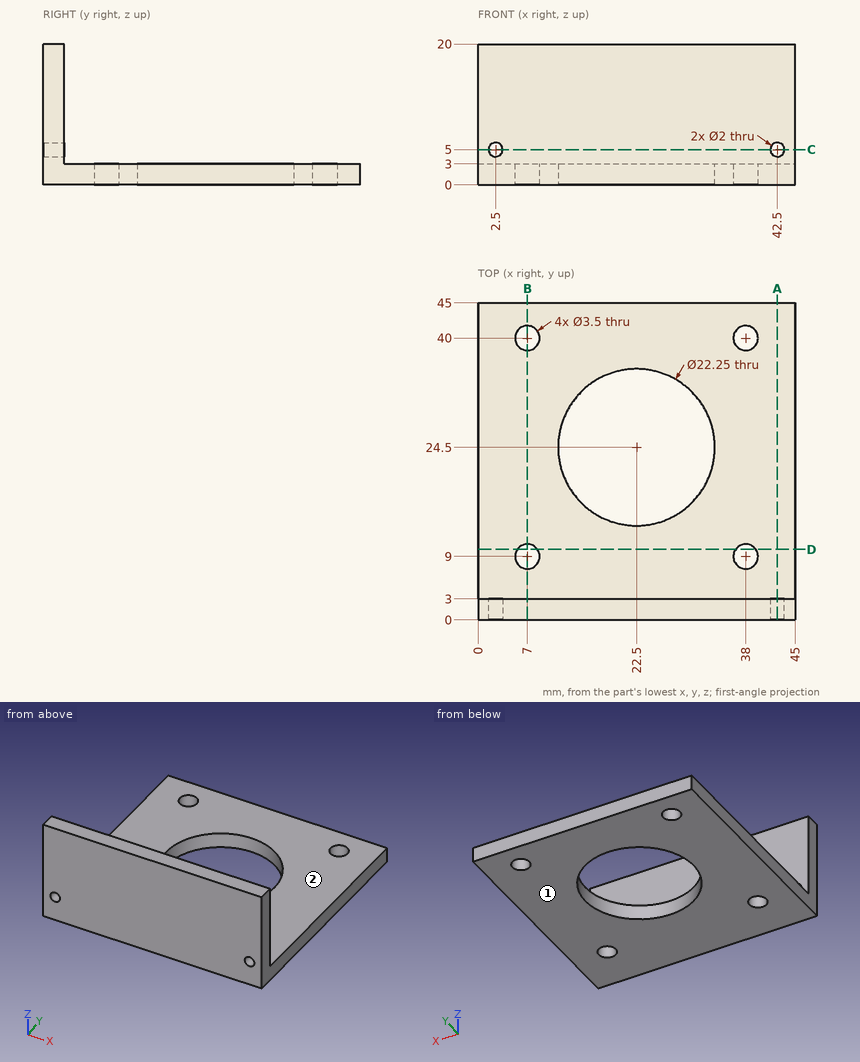
Job drawing, mm, ordinate dimensions from the low corner. One solid piece. A direction names the side the tool comes from. Give positions to 0.01 mm unless a question says otherwise; leave off trailing zeros. Order: outer loops, then holes, each group sorted by start corner. A loop starts at its lowest first (then second) coordinate and runs counter-clockwise, first axis right, second up. Notation, with made-up numbers: (10, -12.75) - (59, -12.75) arc R14 ccw to (59, -4.75) - close; hole circle Ø9 at (37, 24). An arc over 180 degrees is marked (long way). Return JSON: item names as keys, results as strings.
1) Cut at D-D, the plane y = 10. Give the cut face in (x, z).
Geometry says:
{"outline": "(0, 0) - (5.56, 0) - (5.56, 3) - (0, 3) - close; (8.44, 0) - (36.56, 0) - (36.56, 3) - (8.44, 3) - close; (39.44, 0) - (45, 0) - (45, 3) - (39.44, 3) - close"}
2) 3-axis set-ups, long thin cutter, end or side, ignore diameter. For the marked faces 1 and 2: which of +Z, -Z, +X, -X, +Y, -Y reach the whole face in a straight line?
Geometry says:
{"face 1": "-Z, +X, -X, +Y, -Y", "face 2": "+Z, +X, -X, +Y"}
3) Cut at A-A, the plane x = 42.5. Give the cut face in (y, z), plus the area to 3 significant figures.
Geometry says:
{"outline": "(0, 0) - (45, 0) - (45, 3) - (3, 3) - (3, 4) - (0, 4) - close; (0, 6) - (3, 6) - (3, 20) - (0, 20) - close", "area": "180 mm²"}
4) Cut at C-C, the plane z = 5. Give the cut face in (x, y), plus the area to 3 significant figures.
Geometry says:
{"outline": "(0, 0) - (1.5, 0) - (1.5, 3) - (0, 3) - close; (3.5, 0) - (41.5, 0) - (41.5, 3) - (3.5, 3) - close; (43.5, 0) - (45, 0) - (45, 3) - (43.5, 3) - close", "area": "123 mm²"}
5) Probe line 1 (Y direction, x = 7, z = 1.8); line 2 (Z direction, x = 42.5, y = 2.1); line 3 (Y direction, x = 31.5, z = 11.5). List the from-to ranges inside material, lowest first. Write a range as from..to.
Geometry says:
{"line 1": "0..7.25, 10.75..38.25, 41.75..45", "line 2": "0..4, 6..20", "line 3": "0..3"}
6) Cut at B-B, the plane x = 7. Give the cut face in (y, z), plus the area to 3 significant figures.
Geometry says:
{"outline": "(0, 0) - (7.25, 0) - (7.25, 3) - (3, 3) - (3, 20) - (0, 20) - close; (10.75, 0) - (38.25, 0) - (38.25, 3) - (10.75, 3) - close; (41.75, 0) - (45, 0) - (45, 3) - (41.75, 3) - close", "area": "165 mm²"}
7) Flat gauge pins, fed straight in: P1, Ø3, axis at x = 2.5, z = 5, coming from the +Y side; P2, Ø4, axis at x = 38, y = 40, coming from the +Z side. Where does each tip first touch, or does it go through?
Geometry says:
{"P1": "y = 3", "P2": "z = 3"}
